The listing builds one solid part. Answer for the finished solid, in the listing's coordinates (mm). A direction names the side the tool comes from. Round coordinates to 2 decimals unless told otherwise and drop trailing zeros. Loops run counter-clockwise (first coordinate to the right, second up) from the corner with the lowest first, then second, coordinate; pieces in that order, holes last. Notation, with made-up numbers: M 70,67.5 L 107,67.5 A12 ccw 107,72.5 Z; hole C -18.5,8.5 d2. An arc over 180 degrees is marked long. Answer as a JSON object with one key per item and string values.
Autodesk Inventor part; units mm, degrees
ref_plane "YZ Plane" through (0, 0, 0) normal (1, 0, 0) x (0, 1, 0)
ref_plane "XZ Plane" through (0, 0, 0) normal (0, 1, 0) x (-1, 0, 0)
ref_plane "XY Plane" through (0, 0, 0) normal (0, 0, 1) x (1, 0, 0)
sketch "Sketch1" plane through (0, 0, 0) normal (0, 0, 1) x (1, 0, 0)
  line L0 (0, 20) -> (30, 20)
  line L1 (0, 20) -> (0, 0)
  line L2 (-45, 20) -> (-45, 35)
  arc A0 (30, 25) -> (-45, 35) centre (-45, -251.25) ccw
  line L3 (-45, 20) -> (-45, 0)
  line L4 (0, -20) -> (30, -20)
  line L5 (45, -20) -> (45, -20.4834)
  line L6 (0, -20) -> (0, 0)
  line L7 (-45, -20) -> (-45, -35)
  arc A1 (-45, -35) -> (30, -25) centre (-45, 251.25) ccw
  line L8 (-45, -20) -> (-45, 0)
  line L9 (30, 25) -> (30, 20)
  line L10 (30, -25) -> (30, -20)
  point P0 (45, 20.4834)
  point P1 (45, 22.5)
  point P2 (30, 37.5)
  point P3 (-25, -20)
  point P4 (0, -32.987)
  point P5 (45, -22.5)
  point P6 (30, -37.5)
  point P7 (45, -22.5)
  point P8 (30, -37.5)
  dimension "d17" = 15
extrude "Extrusion1" add sketch "Sketch1" along normal mid plane 30
sketch "Sketch3" plane through (0, -20, 15) normal (0, 1, 0) x (1, 0, 0)
  line L0 (0, 0) -> (0, 30)
  line L1 (30, 0) -> (0, 0)
  line L2 (0, 30) -> (30, 30)
  circle A0 centre (36.5, 15) radius 2
  line L3 (30, 30) -> (30, 0)
  point P0 (0, 15)
  dimension "d18" = 4
extrude "Extrusion3" cut sketch "Sketch3" along normal through all both and the other way through all contours A0
fillet "Fillet3" radius 30 1 edges at (30, 25, 0)
fillet "Fillet4" radius 30 1 edges at (30, -25, 0)
sketch "Sketch6" plane through (-45, -35, 15) normal (-1, 0, 0) x (0, 0, 1)
  line L0 (-24.0585, 25.4415) -> (-25, 24.5) construction
  line L1 (-4.3571, 37.8214) -> (-10.3571, 37.8214)
  line L2 (-10.3571, 37.8214) -> (-10.3571, 31.8214)
  line L3 (-10.3571, 31.8214) -> (-4.5, 31.8214)
  line L4 (-25, 37.8214) -> (-19, 37.8214)
  line L5 (-19, 37.8214) -> (-19, 31.8214)
  line L6 (-19, 31.8214) -> (-25, 31.8214)
  line L7 (-25, 24.5) -> (-25, 31.8214)
  line L8 (-25, 37.8214) -> (-25, 45)
  line L9 (-4.3571, 45) -> (-4.3571, 37.8214)
  line L10 (-4.5, 31.8214) -> (-4.5, 24.5)
  line L11 (-11.6786, 45) -> (-11.6786, 39)
  line L12 (-11.6786, 39) -> (-17.6786, 39)
  line L13 (-17.6786, 39) -> (-17.6786, 45)
  line L14 (-25, 45) -> (-17.6786, 45)
  line L15 (-11.6786, 45) -> (-4.3571, 45)
  line L16 (-17.6786, 24.5) -> (-17.6786, 30.5)
  line L17 (-17.6786, 30.5) -> (-11.6786, 30.5)
  line L18 (-11.6786, 30.5) -> (-11.6786, 24.5)
  line L19 (-4.5, 24.5) -> (-11.6786, 24.5)
  line L20 (-17.6786, 24.5) -> (-25, 24.5)
  dimension "d59" = 20.5
  dimension "d67" = 6
  dimension "d68" = 6
  dimension "d69" = 6
  dimension "d70" = 6
  dimension "d71" = 6
  dimension "d73" = 6
extrude "Extrusion5" cut sketch "Sketch6" against normal blind 42
sketch "Sketch7" plane through (-45, -35, 15) normal (-1, 0, 0) x (0, 0, 1)
  line L0 (-30, 50) -> (0, 50)
  line L1 (0, 50) -> (0, 20)
  line L2 (0, 20) -> (-30, 20)
  line L3 (-30, 20) -> (-30, 50)
  line L4 (-30, 50) -> (0, 20) construction
  line L5 (0, 50) -> (-30, 20) construction
  line L6 (-22.5355, 32.4645) -> (-22.5355, 28.5251)
  line L7 (-24.5355, 32.4645) -> (-22.5355, 32.4645)
  line L8 (-24.5355, 25.4645) -> (-24.5355, 32.4645)
  line L9 (-17.5355, 25.4645) -> (-24.5355, 25.4645)
  line L10 (-17.5355, 27.4645) -> (-17.5355, 25.4645)
  line L11 (-21.4749, 27.4645) -> (-17.5355, 27.4645)
  line L12 (-17.9393, 31) -> (-21.4749, 27.4645)
  line L13 (-12.0607, 31) -> (-17.9393, 31)
  line L14 (-8.5251, 27.4645) -> (-12.0607, 31)
  line L15 (-12.4645, 27.4645) -> (-8.5251, 27.4645)
  line L16 (-12.4645, 25.4645) -> (-12.4645, 27.4645)
  line L17 (-5.4645, 25.4645) -> (-12.4645, 25.4645)
  line L18 (-5.4645, 32.4645) -> (-5.4645, 25.4645)
  line L19 (-7.4645, 32.4645) -> (-5.4645, 32.4645)
  line L20 (-7.4645, 28.5251) -> (-7.4645, 32.4645)
  line L21 (-11, 32.0607) -> (-7.4645, 28.5251)
  line L22 (-11, 37.9393) -> (-11, 32.0607)
  line L23 (-7.4645, 41.4749) -> (-11, 37.9393)
  line L24 (-7.4645, 37.5355) -> (-7.4645, 41.4749)
  line L25 (-5.4645, 37.5355) -> (-7.4645, 37.5355)
  line L26 (-5.4645, 44.5355) -> (-5.4645, 37.5355)
  line L27 (-12.4645, 44.5355) -> (-5.4645, 44.5355)
  line L28 (-12.4645, 42.5355) -> (-12.4645, 44.5355)
  line L29 (-8.5251, 42.5355) -> (-12.4645, 42.5355)
  line L30 (-12.0607, 39) -> (-8.5251, 42.5355)
  line L31 (-17.9393, 39) -> (-12.0607, 39)
  line L32 (-21.4749, 42.5355) -> (-17.9393, 39)
  line L33 (-17.5355, 42.5355) -> (-21.4749, 42.5355)
  line L34 (-17.5355, 44.5355) -> (-17.5355, 42.5355)
  line L35 (-24.5355, 44.5355) -> (-17.5355, 44.5355)
  line L36 (-24.5355, 37.5355) -> (-24.5355, 44.5355)
  line L37 (-22.5355, 37.5355) -> (-24.5355, 37.5355)
  line L38 (-22.5355, 41.4749) -> (-22.5355, 37.5355)
  line L39 (-19, 37.9393) -> (-22.5355, 41.4749)
  line L40 (-19, 32.0607) -> (-19, 37.9393)
  line L41 (-22.5355, 28.5251) -> (-19, 32.0607)
  line L42 (-30, 70) -> (0, 70)
  line L43 (-30, 0) -> (-30, 70)
  line L44 (0, 70) -> (0, 0)
  line L45 (-30, 0) -> (0, 0)
  point P0 (-15, 35)
  dimension "d47" = 30
  dimension "d48" = 30
extrude "Extrusion6" cut sketch "Sketch7" against normal blind 30 contours L43 L42 L44 L0 | L0 L1 L2 L3 | L2 L44 L45 L43 | L6 L41 L40 L39 L38 L37 L36 L35 L34 L33 L32 L31 L30 L29 L28 L27 L26 L25 L24 L23 L22 L21 L20 L19 L18 L17 L16 L15 L14 L13 L12 L11 L10 L9 L8 L7
fillet "Fillet5" radius 10 1 edges at (-15, 33.4236, 0)
fillet "Fillet6" radius 10 1 edges at (-15, -33.4236, 0)
sketch "Sketch8" plane through (0, -20, 15) normal (0, 1, 0) x (1, 0, 0)
  line L0 (0, 0) -> (0, 30)
  line L1 (30, 0) -> (0, 0)
  line L2 (0, 30) -> (30, 30)
  circle A0 centre (36.5, 15) radius 2
  arc A1 (37.9617, 6.6266) -> (37.9617, 23.3734) centre (36.5, 15) ccw
  line L3 (0, 0) -> (37.9617, 6.6266)
  line L4 (0, 30) -> (37.9617, 23.3734)
  line L5 (-15, 0) -> (-15, 30)
  line L6 (0, 0) -> (-15, 0)
  line L7 (-15, 0) -> (-15, 30)
  line L8 (-15, 0) -> (-15, 30)
  line L9 (0, 12.4645) -> (0, 5.4645)
  line L10 (-15, 30) -> (0, 30)
  line L11 (-3.552, 30) -> (-3.552, 0)
  line L12 (30, 30) -> (30, 0)
  point P0 (0, 15)
extrude "Extrusion7" cut sketch "Sketch8" along normal through all both and the other way through all contours L6 L11 L10 L0 | L0 L4 L12 L3 | L12 L4 A1 L3 | L6 L5 L10 L11 | A0 keep common part
sketch "Sketch9" plane through (0, -20, 15) normal (0, 1, 0) x (1, 0, 0)
  circle A0 centre (21, 15) radius 4
  line L0 (30, 24.7632) -> (30, 5.2368)
  point P0 (0, 15)
  point P1 (30, 15)
  dimension "d55" = 8
  dimension "d56" = 9
extrude "Extrusion8" cut sketch "Sketch9" along normal through all both and the other way through all
sketch "Sketch10" plane through (-15, -35, 15) normal (-1, 0, 0) x (0, 0, 1)
  point P0 (-15, 35)
sketch "Sketch11" plane through (-15, -35, 15) normal (-1, 0, 0) x (0, 0, 1)
  line L0 (-25, 45) -> (-17.6786, 45)
  line L1 (-4.5, 24.5) -> (-11.6786, 24.5)
  line L2 (-27.75, 22.25) -> (-2.25, 22.25)
  line L3 (-2.25, 22.25) -> (-2.25, 47.75)
  line L4 (-2.25, 47.75) -> (-27.75, 47.75)
  line L5 (-27.75, 47.75) -> (-27.75, 22.25)
  line L6 (-17.6786, 45) -> (-17.6786, 39)
  line L7 (-17.6786, 45) -> (-17.6786, 39)
  line L8 (-17.6786, 39) -> (-11.6786, 39)
  line L9 (-17.6786, 39) -> (-11.6786, 39)
  line L10 (-11.6786, 39) -> (-11.6786, 45)
  line L11 (-11.6786, 39) -> (-11.6786, 45)
  line L12 (-10.3571, 37.8214) -> (-4.3571, 37.8214)
  line L13 (-4.3571, 37.8214) -> (-10.3571, 37.8214)
  line L14 (-10.3571, 37.8214) -> (-10.3571, 31.8214)
  line L15 (-10.3571, 37.8214) -> (-10.3571, 31.8214)
  line L16 (-4.5, 31.8214) -> (-10.3571, 31.8214)
  line L17 (-10.3571, 31.8214) -> (-4.5, 31.8214)
  line L18 (-11.6786, 30.5) -> (-11.6786, 24.5)
  line L19 (-11.6786, 24.5) -> (-11.6786, 30.5)
  line L20 (-17.6786, 30.5) -> (-11.6786, 30.5)
  line L21 (-11.6786, 30.5) -> (-17.6786, 30.5)
  line L22 (-17.6786, 30.5) -> (-17.6786, 24.5)
  line L23 (-17.6786, 30.5) -> (-17.6786, 24.5)
  line L24 (-19, 37.8214) -> (-25, 37.8214)
  line L25 (-25, 37.8214) -> (-19, 37.8214)
  line L26 (-25, 31.8214) -> (-19, 31.8214)
  line L27 (-19, 37.8214) -> (-19, 31.8214)
  line L28 (-19, 31.8214) -> (-25, 31.8214)
  line L29 (-25, 45) -> (-17.6786, 45)
  line L30 (-11.6786, 45) -> (-4.5, 45)
  line L31 (-25, 24.5) -> (-25, 31.8214)
  line L32 (-25, 37.8214) -> (-25, 45)
  line L33 (-4.5, 24.5) -> (-11.6786, 24.5)
  line L34 (-17.6786, 24.5) -> (-25, 24.5)
  line L35 (-4.5, 45) -> (-4.5, 37.8214)
  line L36 (-4.5, 31.8214) -> (-4.5, 24.5)
  point P0 (-15, 35)
extrude "Extrusion9" add sketch "Sketch11" along normal blind 45
sketch "Sketch12" plane through (-60, -35, 15) normal (-1, 0, 0) x (0, 0, 1)
  line L0 (-17.6786, 45) -> (-17.6786, 39)
  line L1 (-17.6786, 45) -> (-17.6786, 39)
  line L2 (-17.6786, 39) -> (-11.6786, 39)
  line L3 (-17.6786, 39) -> (-11.6786, 39)
  line L4 (-11.6786, 39) -> (-11.6786, 45)
  line L5 (-11.6786, 39) -> (-11.6786, 45)
  line L6 (-11.6786, 45) -> (-17.6786, 45)
  line L7 (-11.6786, 30.5) -> (-17.6786, 30.5)
  line L8 (-17.6786, 30.5) -> (-11.6786, 30.5)
  line L9 (-11.6786, 24.5) -> (-11.6786, 30.5)
  line L10 (-11.6786, 30.5) -> (-11.6786, 24.5)
  line L11 (-17.6786, 24.5) -> (-25, 24.5)
  line L12 (-11.6786, 24.5) -> (-17.6786, 24.5)
  line L13 (-17.6786, 24.5) -> (-17.6786, 30.5)
  point P0 (-15, 35)
extrude "Extrusion10" cut sketch "Sketch12" against normal up to surface (57 mm away)
sketch "Sketch13" plane through (-15, 12.75, 12.75) normal (0, 1, 0) x (1, 0, 0)
  point P0 (15, 12.75)
sketch "Sketch15" plane through (-15, -12.75, -12.75) normal (0, 0, -1) x (-1, 0, 0)
  line L0 (0, 25.5) -> (45, 25.5)
  line L1 (41.4, 35.7) -> (45, 35.7)
  arc A0 (41.4, 35.7) -> (41.4, 25.5) centre (45.352, 30.6) ccw
  line L2 (48.6, 35.7) -> (45, 35.7)
  arc A1 (48.6, 25.5) -> (48.6, 35.7) centre (44.648, 30.6) ccw
  line L3 (0, 25.5) -> (45, 25.5)
  line L4 (0, 22.75) -> (45, 22.75)
  line L5 (45, 37.7) -> (36.9, 37.7)
  line L6 (36.9, 37.7) -> (36.9, 25.5)
  line L7 (45, 37.7) -> (53.1, 37.7)
  line L8 (53.1, 37.7) -> (53.1, 25.5)
  line L9 (36.9, 25.5) -> (41.4, 25.5)
  line L10 (48.6, 25.5) -> (53.1, 25.5)
  line L11 (45, 0) -> (45, 25.5)
  point P0 (-15, 12.75)
  point P1 (38.9, 25.5)
  point P2 (38.9, 35.7)
  point P3 (51.1, 25.5)
  point P4 (51.1, 35.7)
  dimension "d85" = 10.2
extrude "Extrusion12" add sketch "Sketch15" against normal blind 15
sketch "Sketch16" plane through (-60, -35, 15) normal (-1, 0, 0) x (0, 0, 1)
  line L0 (-4.5, 24.5) -> (-25, 24.5)
  line L1 (-25, 24.5) -> (-25, 31.8214)
  line L2 (-25, 31.8214) -> (-19, 31.8214)
  line L3 (-19, 31.8214) -> (-19, 37.8214)
  line L4 (-19, 37.8214) -> (-25, 37.8214)
  line L5 (-25, 37.8214) -> (-25, 45)
  line L6 (-25, 45) -> (-4.5, 45)
  line L7 (-4.5, 45) -> (-4.5, 37.8214)
  line L8 (-4.5, 37.8214) -> (-10.3571, 37.8214)
  line L9 (-10.3571, 37.8214) -> (-10.3571, 31.8214)
  line L10 (-10.3571, 31.8214) -> (-4.5, 31.8214)
  line L11 (-4.5, 31.8214) -> (-4.5, 24.5)
  line L12 (-2.25, 22.25) -> (-2.25, 47.75)
  line L13 (-2.25, 47.75) -> (-27.75, 47.75)
  line L14 (-27.75, 47.75) -> (-27.75, 22.25)
  line L15 (-27.75, 22.25) -> (-2.25, 22.25)
  point P0 (-15, 35)
extrude "Extrusion13" add sketch "Sketch16" along normal blind 15
sketch "Sketch17" plane through (-15, 12.75, 12.75) normal (0, 1, 0) x (1, 0, 0)
  circle A0 centre (-56.5, 12.75) radius 2.5
  line L0 (-60, 0) -> (-60, 25.5)
  point P0 (15, 12.75)
  dimension "d96" = 5
  dimension "d97" = 3.5
extrude "Extrusion14" cut sketch "Sketch17" against normal through all
properties part number "Nuckle"
Item 1: The part is cut by section D-D (x = 21). Give the vertices of the cut face in (y, z), then the cut area to 3 significant figures.
Values follow:
{"outline": "M -26.54,-11.33 L -20,-11.33 L -20,-4 L -26.54,-4 Z; M -26.54,4 L -20,4 L -20,11.33 L -26.54,11.33 Z; M 20,-11.33 L 26.54,-11.33 L 26.54,-4 L 20,-4 Z; M 20,4 L 26.54,4 L 26.54,11.33 L 20,11.33 Z", "area": "192 mm^2"}
Item 2: Flat-ended cylindrical pins translate along their axes: P1, Ø8, axis at x = -47, z = 4, coming from the +Y side; P2, Ø16.5, axis at x = -49, z = 4, coming from the -Y side; P3, Ø6.5, axis at x = 21, z = 0, coming from the +Y side; P4, Ø3.5, axis at y = 19.5, z = -8.5, coming from the -X side. Find the tip coordinate at first contact, or state that the pin passes through.
Values follow:
{"P1": "y = 12.75", "P2": "y = -12.75", "P3": "through", "P4": "x = -68.1"}
Item 3: The part is cut by section A-A (x = -71.5). Give the vertices of the cut face in (y, z).
Values follow:
{"outline": "M -12.75,-12.75 L 12.75,-12.75 L 12.75,-2.5 L 10,-2.5 L 10,-10 L 2.82,-10 L 2.82,-4 L -3.18,-4 L -3.18,-10 L -10.5,-10 L -10.5,-2.5 L -12.75,-2.5 Z; M -12.75,2.5 L -10.5,2.5 L -10.5,10.5 L -3.18,10.5 L -3.18,4.64 L 2.82,4.64 L 2.82,10.5 L 10,10.5 L 10,2.5 L 12.75,2.5 L 12.75,12.75 L -12.75,12.75 Z"}
Item 4: Straight lines are drawn through the part: line 1 (Y direction, x = -42, z = 6.5); line 2 (X direction, y = -11, z = 0); line 3 (Y direction, x = -9.5, z = -6.5). For each, find the intervals that lie inside material, in ascending order.
Values follow:
{"line 1": "-12.75 to -10.5, -3.18 to 2.82, 10 to 12.75", "line 2": "-75 to -74, -69 to 0", "line 3": "-31.02 to -10.5, -3.18 to 2.82, 10 to 31.02"}
Item 5: The part is cut by section B-B (y = -4.5). Give the vertices of the cut face in (x, z), then the cut area to 3 significant figures.
Values follow:
{"outline": "M -75,-12.75 L -15,-12.75 L -15,-15 L 0,-15 L 0,15 L -15,15 L -15,12.75 L -75,12.75 L -75,10.5 L -3,10.5 L -3,-10 L -75,-10 Z", "area": "504 mm^2"}
Item 6: Determine the mould class of faces 1 (the face through (-45, -12.75, 0)), 2 (the face through (11.46, -24.53, 13)), 3 (the face through (17, -23, 0)), 4 (the face through (-45, 12.75, 0)) for opening direction X: released by +X, released by -X, zero draft, split by the parting line, or undercut.
Values follow:
{"face 1": "zero draft", "face 2": "released by +X", "face 3": "undercut", "face 4": "undercut"}
Item 7: Which of the six approach directions +Z, -Z, +X, -X, +Y, -Y give full straight-line access (tool end or side, diameter ignored) to faces 5 (the face through (-45, 2, -12.75)), 6 (the face through (-51.9, 19, -5)), 7 (the face through (-53.9, 17.9, -5.4))?
Values follow:
{"face 5": "-Z, -X, +Y, -Y", "face 6": "+Z, -Z, +Y", "face 7": "+Z, -Z"}
